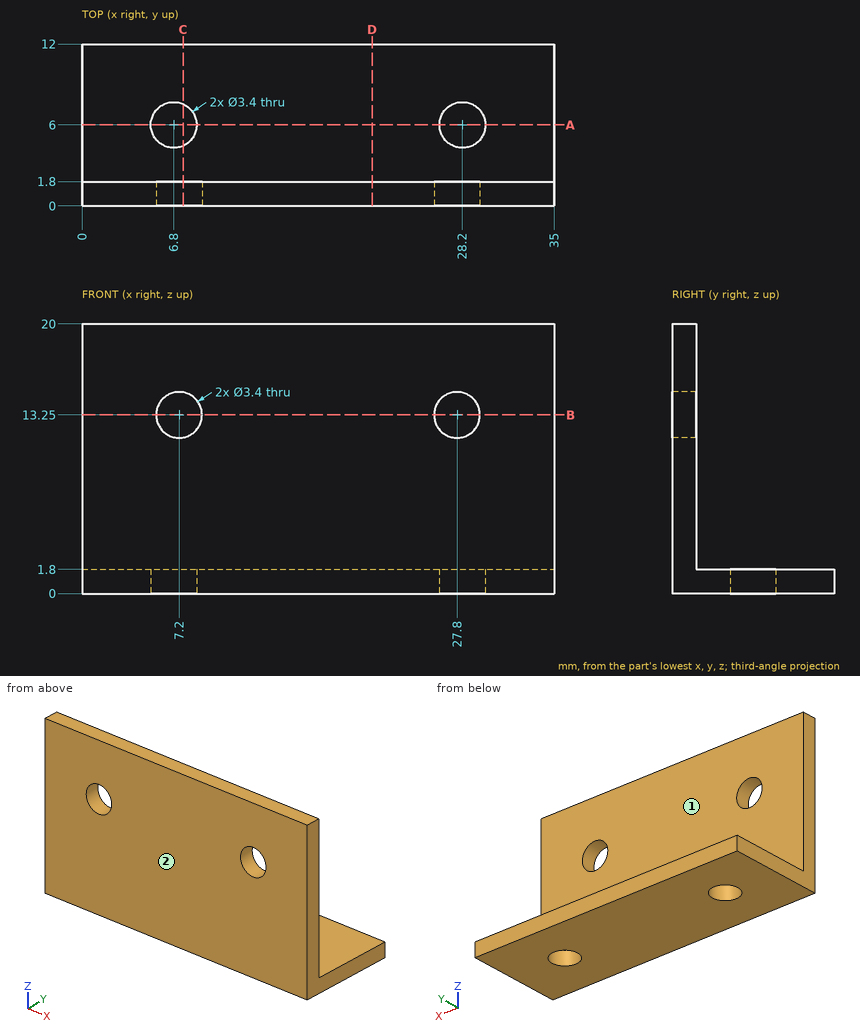
Design review of the part shown in the three views and the two pictorial views. Dimensions are in mm from the part's minimum x, y and z. A direction names the side the tool comes from. Coordinates: 2 decimals unless noted, no trailing zeros. Loops run counter-clockwise (first coordinate to the right, second up) from the corner with the lowest first, then second, coordinate; pieces in that order, holes last.
(1) Consider section D-D, the plane x = 21.5. Give the boundary of the cut face in (y, z).
Determined:
outline: (0, 0) - (12, 0) - (12, 1.8) - (1.8, 1.8) - (1.8, 20) - (0, 20) - close
(2) Tool access review of the marked faces 1 and 2: name each direction out of +Z, -Z, +X, -X, +Y, -Y from which nothing blocks a thin tool from reaching the whole face with its end or side.
Determined:
face 1: +Z, +X, -X, +Y
face 2: +Z, -Z, +X, -X, -Y
(3) Wall thickness on L1, parallel to X at y = 0.9, z = 13.25; L2, parallel to Z at x = 27.8, y = 0.6; L3, parallel to Y at x = 3, z = 10.25: over which ranges is each line inside the solid? List them lowest first.
Determined:
L1: x = 0 to 5.5, 8.9 to 26.1, 29.5 to 35
L2: z = 0 to 11.55, 14.95 to 20
L3: y = 0 to 1.8
(4) Consider section A-A, the plane y = 6. Give the boundary of the cut face in (x, z), plus the area to 3 significant figures.
Determined:
outline: (0, 0) - (5.1, 0) - (5.1, 1.8) - (0, 1.8) - close; (8.5, 0) - (26.5, 0) - (26.5, 1.8) - (8.5, 1.8) - close; (29.9, 0) - (35, 0) - (35, 1.8) - (29.9, 1.8) - close
area: 50.8 mm2
(5) Insertion check: P1, Ø9, axis at x = 17.5, z = 14.5, coming from the +Y side; P2, Ø4.5, axis at x = 28.2, y = 6, coming from the +Z side. Each pin has a flat end and moves straight along its axis. Give the tip position at first contact, or say it passes through.
Determined:
P1: stops at y = 1.8
P2: stops at z = 1.8
(6) Consider section C-C, the plane x = 7.5. Give the boundary of the cut face in (y, z).
Determined:
outline: (0, 0) - (4.45, 0) - (4.45, 1.8) - (1.8, 1.8) - (1.8, 11.58) - (0, 11.58) - close; (0, 14.92) - (1.8, 14.92) - (1.8, 20) - (0, 20) - close; (7.55, 0) - (12, 0) - (12, 1.8) - (7.55, 1.8) - close
(7) Consider section B-B, the plane z = 13.25. Give the boundary of the cut face in (x, y), plus the area to 3 significant figures.
Determined:
outline: (0, 0) - (5.5, 0) - (5.5, 1.8) - (0, 1.8) - close; (8.9, 0) - (26.1, 0) - (26.1, 1.8) - (8.9, 1.8) - close; (29.5, 0) - (35, 0) - (35, 1.8) - (29.5, 1.8) - close
area: 50.8 mm2
